Design review of the part built by this model. Coordinates are the model's own, in mm. Round coordinates to 2 decimals unless told otherwise and drop trailing zeros. Loops run counter-clockwise (first coordinate to the right, second up) from the corner with the lowest first, then second, coordinate; pieces in that order, holes last. Notation, with made-up numbers: (63, 10) - (80, 10) arc R17 ccw to (80, 28) - close; hole circle Ø8 at (-14.5, -23). An arc over 180 degrees is marked (long way). Use one line per item in the form item = value. Start each with the question number.
(1) For pin 1 (1.5 mm diameter, centred on y = 9, z = -64.5, fed in from -X); pin 2 (3 mm diameter, centred on y = 10.5, z = -47.5, fed in from +X), all flat-tipped, find the tip position at first contact; note any pin that passes through.
(2) Wall thickness on probe 1 along X at (y, z) = (1.25, -35); probe 2 along Z at (x, y) = (381.5, 1.75) (3 decimals): over which ranges is each line inside the solid? List them lowest first. Write a range as [from, to].
(3) We need section A-A, the plane z = -39.5. Write out the cut boundary in (x, y).
from build123d import *

# Parameters (mm, degrees)
SKETCH1_W           = 388.62
SKETCH1_H           = 121.92
BOSS_EXTRUDE1_DEPTH = 12.7
SKETCH3_W           = 12.7
SKETCH3_H           = 25.4
TABS_DEPTH          = 12.7
SKETCH4_W           = 5.4
SKETCH4_H           = 12.7
SCREW_SLOT_DEPTH    = 12.7
SKETCH5_W           = 4.1
SKETCH5_H           = 8.15
NUT_SLOT_DEPTH      = 12.7


with BuildPart() as part:
    # Sketch1 → Boss-Extrude1 (new body)
    with BuildSketch(Plane(origin=(0, 0, 0), x_dir=(1, 0, 0), z_dir=(0, 1, 0))):
        with Locations((194.31, 60.96)):
            Rectangle(SKETCH1_W, SKETCH1_H)
    extrude(amount=BOSS_EXTRUDE1_DEPTH)

    # Sketch3 → tabs (add)
    with BuildSketch(Plane(origin=(0, 12.7, 0), x_dir=(1, 0, 0), z_dir=(0, 1, 0))):
        with Locations((-6.35, 109.22)):
            Rectangle(SKETCH3_W, SKETCH3_H)
        with Locations((-6.35, 12.7)):
            Rectangle(SKETCH3_W, SKETCH3_H)
        with Locations((394.97, 12.7)):
            Rectangle(SKETCH3_W, SKETCH3_H)
        with Locations((394.97, 109.22)):
            Rectangle(SKETCH3_W, SKETCH3_H)
    extrude(amount=-TABS_DEPTH)

    # Sketch4 → screw slot (cut)
    with BuildSketch(Plane.ZY):
        with Locations((-60.96, 6.35)):
            Rectangle(SKETCH4_W, SKETCH4_H)
    screw_slot = extrude(amount=-SCREW_SLOT_DEPTH, mode=Mode.SUBTRACT)

    # Sketch5 → nut slot (cut)
    with BuildSketch(Plane(origin=(0, 12.7, 0), x_dir=(1, 0, 0), z_dir=(0, 1, 0))):
        with Locations((8, 60.96)):
            Rectangle(SKETCH5_W, SKETCH5_H)
    nut_slot = extrude(amount=-NUT_SLOT_DEPTH, mode=Mode.SUBTRACT)

    # Mirror1: screw slot, nut slot across plane
    add(screw_slot.mirror(Plane(origin=(194.31, 0, 0), x_dir=(0, 0, 1), z_dir=(1, 0, 0))), mode=Mode.SUBTRACT)
    add(nut_slot.mirror(Plane(origin=(194.31, 0, 0), x_dir=(0, 0, 1), z_dir=(1, 0, 0))), mode=Mode.SUBTRACT)


solid = part.part
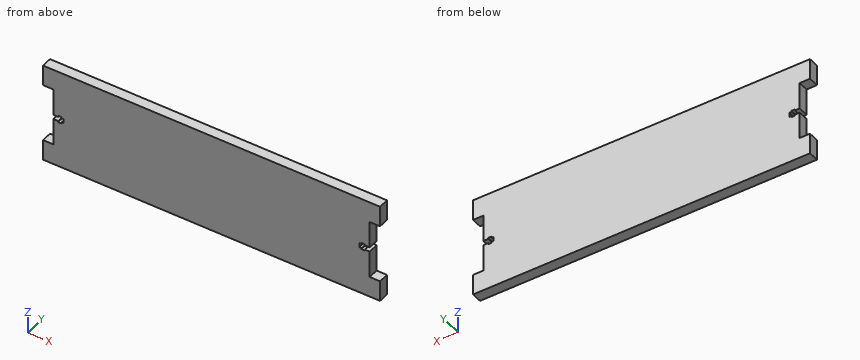
Data:
q1.pin_1 = 0
q1.pin_2 = 388.62
q2.probe_1 = [0, 388.62]
q2.probe_2 = [-121.92, -65.035], [-56.885, 0]
q3.outline = (0, 0) - (388.62, 0) - (388.62, 12.7) - (0, 12.7) - close
